```python
from build123d import *

# Parameters (mm, degrees)
F1_DEPTH = 19
F2_R     = 5
F3_R     = 2
F4_R     = 5
F5_SIZE  = 1


with BuildPart() as f1:
    # F0 (on Top) → F1 (new body)
    with BuildSketch(Plane.XY):
        Polygon((3, 0), (0, 0), (0, -15), (21.13954, -1.653846), (21.13954, 43.346154), (40.63954, 43.346154), (40.63954, 23.346154), (43.63954, 23.346154), (43.63954, 46.346154), (18.13954, 46.346154), (18.13954, 0), (3, -9.558138), align=None)
    extrude(amount=F1_DEPTH)

    # F2
    f2_edges = [f1.edges().sort_by_distance(p)[0] for p in [
        (1.5, 0, 0),
        (1.5, 0, 19),
    ]]
    fillet(f2_edges, radius=F2_R)

    # F3
    f3_edges = [f1.edges().sort_by_distance(p)[0] for p in [
        (18.13954, 46.346154, 9.5),
        (3, -9.558138, 9.5),
        (43.63954, 23.346154, 9.5),
        (18.13954, 0, 9.5),
        (21.13954, -1.653846, 9.5),
        (43.63954, 46.346154, 9.5),
    ]]
    fillet(f3_edges, radius=F3_R)

    # F4
    f4_edges = [f1.edges().sort_by_distance(p)[0] for p in [
        (0, -15, 9.5),
    ]]
    fillet(f4_edges, radius=F4_R)

    # F5
    f5_edges = [f1.edges().sort_by_distance(p)[0] for p in [
        (13.938232, -6.200292, 19),
        (11.637462, -4.104996, 19),
        (30.88954, 43.346154, 0),
        (40.63954, 33.346154, 0),
        (30.88954, 43.346154, 19),
        (40.63954, 33.346154, 19),
    ]]
    chamfer(f5_edges, length=F5_SIZE)


solid = f1.part
```
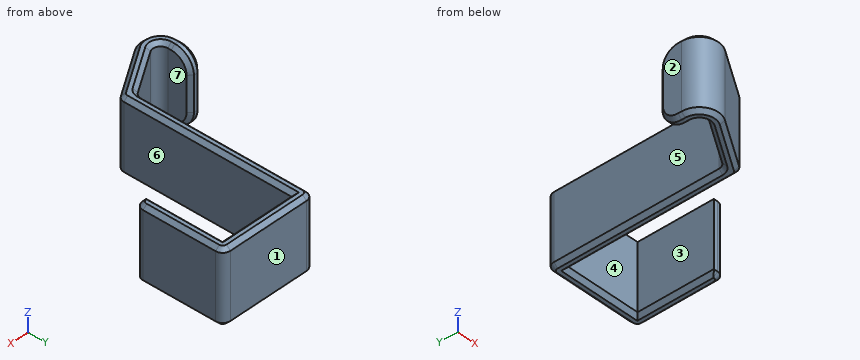
The listing builds one solid part. Answer for the finished solid, in the listing's coordinates (mm). Face numbers are marked on the shaded views. A direction names the side the tool comes from. Coordinates: 2 decimals unless noted, no trailing zeros. Write each loop counter-clockwise with the first axis right and the second up, starting at its lowest first coordinate (ties: lowest second). Pieces come first, ordered by that corner, then holes. Notation, with made-up numbers: (-37, 18.25) - (-20, 18.25) arc R14 ccw to (-20, 29.25) - close; hole circle Ø10 at (40, 4). An arc over 180 degrees is marked (long way). Return JSON: item names as keys, results as strings. Group by question number.
Q1. Which of the six approach directions +Z, -Z, +X, -X, +Y, -Y give full straight-line access (tool end or side, diameter ignored) to the marked faces 5, 6 and 7?
Q2. The part is cut by section A-A on y = 29. Write down the section's boundary in (x, z), and give its area (3 significant figures).
Q3. Find the intervals of material crossed by line 1 along X through (y, z) = (40.5, 5.5); line 2 along Y through (x, z) = (26, 3.75); line 3 along X through (y, z) = (18.5, 13.75), in increasing order. Write a range as [from, to].
Q4. The part is cut by section C-C on y = 22.5. Write down the section's boundary in (x, z), and give its area (3 significant figures).
Q5. The part is cut by section B-B on x = 26. Write down the section's boundary in (y, z), and give its area (3 significant figures).
Q6. Flat-ended cylindrical pins translate along their axes: pin 1 Ø5 at (y, z) = (25.5, 11.5) entering from -X; pin 2 Ø4 at (y, z) = (-3.5, 7.5) entering from +X; pin 3 Ø8.5 at (y, z) = (12.5, 13) entering from +X. Find the tip coordinate at first contact, or state that the pin passes through.
Q7. For a pull along X with two mould halves and no side action, classify the marked faces 1, 2, 3 and 4 as +X half, -X half, draft (parallel to the pull), parting line (faces both ways), or undercut.
Evaluation:
{
 "1": {"face 5": "+Z, -Z, -X, +Y", "face 6": "+Z, -Z, -Y", "face 7": "+Z, -Z, +Y"},
 "2": {"outline": "(18.14, 1) - (19.14, 0) - (20.14, 0) - (21.14, 1) - (21.14, 18) - (20.14, 19) - (19.14, 19) - (18.14, 18) - close; (40.64, 1) - (41.64, 0) - (42.64, 0) - (43.64, 1) - (43.64, 18) - (42.64, 19) - (41.64, 19) - (40.64, 18) - close", "area": "110 mm2"},
 "3": {"line 1": "x = [18.14, 21.14], [40.64, 43.64]", "line 2": "y = [43.35, 46.35]", "line 3": "x = [18.14, 21.14]"},
 "4": {"outline": "(18.14, 1) - (19.14, 0) - (20.14, 0) - (21.14, 1) - (21.14, 18) - (20.14, 19) - (19.14, 19) - (18.14, 18) - close", "area": "55.0 mm2"},
 "5": {"outline": "(43.35, 1) - (44.35, 0) - (45.35, 0) - (46.35, 1) - (46.35, 18) - (45.35, 19) - (44.35, 19) - (43.35, 18) - close", "area": "55.0 mm2"},
 "6": {"pin 1": "stops at x = 18.14", "pin 2": "stops at x = 20.9", "pin 3": "stops at x = 21.14"},
 "7": {"face 1": "draft", "face 2": "-X half", "face 3": "undercut", "face 4": "undercut"}
}
